```python
from build123d import *

# Parameters (mm, degrees)
BOSS_EXTRUDE2_DEPTH = 4


with BuildPart() as part:
    # Sketch1 → Boss-Extrude2 (new body)
    with BuildSketch(Plane.XY):
        Polygon((-73.597643579, 117.281365478), (67.863251178, 117.281365478), (104.632803799, 80.511812856), (104.632803799, -60.949081901), (67.894125273, -97.50252168), (-73.566769484, -97.50252168), (-110.367196201, -60.702096755), (-110.367196201, 80.511812856), align=None)
        with BuildLine():
            Line((-47.610288665, 70.602021163), (41.576775637, 70.602021163))
            ThreePointArc((41.576775637, 70.602021163), (50.108558427, 62.070238373), (41.576775637, 53.538455583))
            Line((41.576775637, 53.538455583), (-47.610288665, 53.538455583))
            ThreePointArc((-47.610288665, 53.538455583), (-56.142071455, 62.070238373), (-47.610288665, 70.602021163))
        make_face(mode=Mode.SUBTRACT)
        with BuildLine():
            Line((-47.610288665, -50.792305062), (41.576775637, -50.792305062))
            ThreePointArc((41.576775637, -50.792305062), (50.108558427, -42.260522272), (41.576775637, -33.728739482))
            Line((41.576775637, -33.728739482), (-47.610288665, -33.728739482))
            ThreePointArc((-47.610288665, -33.728739482), (-56.142071455, -42.260522272), (-47.610288665, -50.792305062))
        make_face(mode=Mode.SUBTRACT)
        with BuildLine():
            Line((-58.385806079, -20.095141949), (-58.385806079, 39.904858051))
            ThreePointArc((-58.385806079, 39.904858051), (-50.403357017, 47.887307113), (-42.420907955, 39.904858051))
            Line((-42.420907955, 39.904858051), (-42.420907955, -20.095141949))
            ThreePointArc((-42.420907955, -20.095141949), (-50.403357017, -28.077591011), (-58.385806079, -20.095141949))
        make_face(mode=Mode.SUBTRACT)
        with BuildLine():
            Line((-43.951300834, 90.135788358), (-43.951300834, 107.780882998))
            ThreePointArc((-43.951300834, 107.780882998), (-41.951300834, 109.780882998), (-39.951300834, 107.780882998))
            Line((-39.951300834, 107.780882998), (-39.951300834, 90.135788358))
            ThreePointArc((-39.951300834, 90.135788358), (-41.951300834, 88.135788358), (-43.951300834, 90.135788358))
        make_face(mode=Mode.SUBTRACT)
        with BuildLine():
            Line((39.83957888, 89.970561723), (39.910868679, 107.61551235))
            ThreePointArc((39.910868679, 107.61551235), (37.918965413, 109.623576437), (35.910901326, 107.63167317))
            Line((35.910901326, 107.63167317), (35.839611526, 89.986722543))
            ThreePointArc((35.839611526, 89.986722543), (37.831514793, 87.978658457), (39.83957888, 89.970561723))
        make_face(mode=Mode.SUBTRACT)
        with BuildLine():
            Line((-83.098126059, -33.179247031), (-100.743220699, -33.179247031))
            ThreePointArc((-100.743220699, -33.179247031), (-102.743220699, -31.179247031), (-100.743220699, -29.179247031))
            Line((-100.743220699, -29.179247031), (-83.098126059, -29.179247031))
            ThreePointArc((-83.098126059, -29.179247031), (-81.098126059, -31.179247031), (-83.098126059, -33.179247031))
        make_face(mode=Mode.SUBTRACT)
        with BuildLine():
            Line((-82.932899424, 50.611632682), (-100.577850051, 50.682922481))
            ThreePointArc((-100.577850051, 50.682922481), (-102.585914138, 48.691019215), (-100.594010871, 46.682955128))
            Line((-100.594010871, 46.682955128), (-82.949060244, 46.611665329))
            ThreePointArc((-82.949060244, 46.611665329), (-80.940996157, 48.603568595), (-82.932899424, 50.611632682))
        make_face(mode=Mode.SUBTRACT)
        with BuildLine():
            Line((40.21690933, -72.326072256), (40.21690933, -89.971166897))
            ThreePointArc((40.21690933, -89.971166897), (38.21690933, -91.971166897), (36.21690933, -89.971166897))
            Line((36.21690933, -89.971166897), (36.21690933, -72.326072256))
            ThreePointArc((36.21690933, -72.326072256), (38.21690933, -70.326072256), (40.21690933, -72.326072256))
        make_face(mode=Mode.SUBTRACT)
        with BuildLine():
            Line((-43.573970383, -72.160845622), (-43.645260182, -89.805796249))
            ThreePointArc((-43.645260182, -89.805796249), (-41.653356916, -91.813860335), (-39.645292829, -89.821957069))
            Line((-39.645292829, -89.821957069), (-39.574003029, -72.177006442))
            ThreePointArc((-39.574003029, -72.177006442), (-41.565906296, -70.168942355), (-43.573970383, -72.160845622))
        make_face(mode=Mode.SUBTRACT)
        with BuildLine():
            Line((79.363734556, 50.988963133), (97.008829196, 50.988963133))
            ThreePointArc((97.008829196, 50.988963133), (99.008829196, 48.988963133), (97.008829196, 46.988963133))
            Line((97.008829196, 46.988963133), (79.363734556, 46.988963133))
            ThreePointArc((79.363734556, 46.988963133), (77.363734556, 48.988963133), (79.363734556, 50.988963133))
        make_face(mode=Mode.SUBTRACT)
        with BuildLine():
            Line((79.198507921, -32.801916581), (96.843458548, -32.87320638))
            ThreePointArc((96.843458548, -32.87320638), (98.851522635, -30.881303113), (96.859619368, -28.873239027))
            Line((96.859619368, -28.873239027), (79.214668741, -28.801949227))
            ThreePointArc((79.214668741, -28.801949227), (77.206604654, -30.793852494), (79.198507921, -32.801916581))
        make_face(mode=Mode.SUBTRACT)
    extrude(amount=BOSS_EXTRUDE2_DEPTH)


solid = part.part
```
The listing builds one solid part. Answer for the finished solid, in the listing's coordinates (mm). A direction names the side the tool comes from. Coordinates: 2 decimals unless noted, no trailing zeros. Loops run counter-clockwise (first coordinate to the right, second up) from the corner with the lowest first, then second, coordinate; pieces in that order, holes last. Notation, with made-up numbers: M 43,35 L 94,35 A23 ccw 94,61 Z; hole C 79.25,-27 d11. An arc over 180 degrees is marked long. Answer as a JSON object with one key per item and string values. Group by question number.
Item 1: Consider L1, parallel to Y at x = -28.5, z = 3; L2, parallel to Y at x = 94, z = 0.35; L3, parallel to X at y = 106.5, z = 1.5. Determine where each line is inside the solid, lowest interval first.
Item 2: Which of the six approach directions +Z, -Z, +X, -X, +Y, -Y give full straight-line access (tool end or side, diameter ignored) to faces 4 (the face through (86.52, -78.97, 1.97)), 5 (the face through (50.106, 62.258, 1.972))?
Item 3: Section B-B (y = 21.5) is taken. Write down the section's boundary in (x, z).
Item 4: Section C-C (y = -75) is taken. Write down the section's boundary in (x, z), and give its area (3 significant figures).
Item 5: Section D-D (z = 0.75) is taken. Give the number of separate pieces and of enclosed holes in the cut face, and give its area (3 significant figures).
Item 6: Section A-A (x = 88.5) is taken. Write down the section's boundary in (y, z), and give its area (3 significant figures).
Item 7: Each of these flat-tipped pins is pushed along its axis until it touches: P1, Ø1.2, axis at y = 99.5, z = 3, coming from the +X side; P2, Ø5, axis at x = -28.5, y = -76, coming from the -Z side; P3, Ø2, axis at y = -78.5, z = 2.5, coming from the -X side. Where does it stop, or does it pass through?
Item 8: Determine the mould class of faces 1 (the face through (-1, 11, 0)), 2 (the face through (-92.24, 98.64, 1.97)), 3 (the face through (-56.14, -42.07, 1.97)) for opening direction X: +X half, -X half, draft (parallel to the pull), parting line (faces both ways), or undercut.
Solved:
{
 "1": {"L1": "y = -97.5 to -50.79, -33.73 to 53.54, 70.6 to 117.28", "L2": "y = -71.53 to -32.86, -28.86 to 46.99, 50.99 to 91.14", "L3": "x = -84.38 to -43.95, -39.95 to 35.91, 39.91 to 78.64"},
 "2": {"face 4": "+Z, -Z, +X, -Y", "face 5": "+Z, -Z"},
 "3": {"outline": "M -110.37,0 L -58.39,0 L -58.39,4 L -110.37,4 Z; M -42.42,0 L 104.63,0 L 104.63,4 L -42.42,4 Z"},
 "4": {"outline": "M -96.07,0 L -43.59,0 L -43.59,4 L -96.07,4 Z; M -39.59,0 L 36.22,0 L 36.22,4 L -39.59,4 Z; M 40.22,0 L 90.51,0 L 90.51,4 L 40.22,4 Z", "area": "714 mm2"},
 "5": {"separate pieces": "1", "enclosed holes": "11", "area": "38,200 mm2"},
 "6": {"outline": "M -77,0 L -32.84,0 L -32.84,4 L -77,4 Z; M -28.84,0 L 46.99,0 L 46.99,4 L -28.84,4 Z; M 50.99,0 L 96.64,0 L 96.64,4 L 50.99,4 Z", "area": "663 mm2"},
 "7": {"P1": "stops at x = 86.24", "P2": "stops at z = 0", "P3": "stops at x = -93.57"},
 "8": {"face 1": "draft", "face 2": "-X half", "face 3": "undercut"}
}
